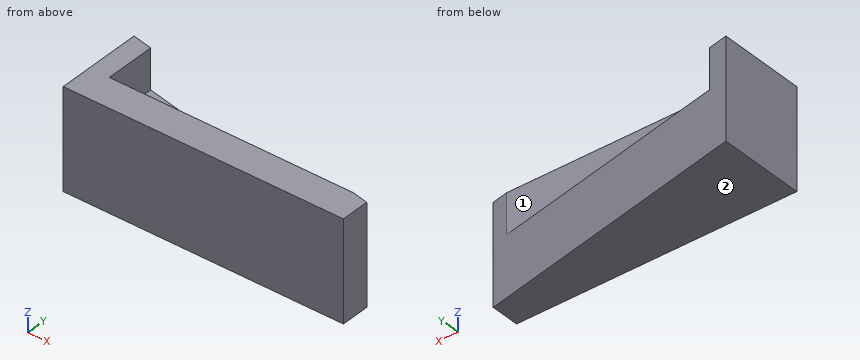
from build123d import *

# Parameters (mm, degrees)
F1_DEPTH = 15
F3_DEPTH = 10
F6_DEPTH = 3
F8_DEPTH = 25


with BuildPart() as f1:
    # F0 (on Top) → F1 (new body)
    with BuildSketch(Plane.XY):
        Polygon((60, 12.5), (0, 0), (60, 0), align=None)
        Polygon((60, 12.5), (60, 0), (90, 0), (90, 18.75), align=None)
    extrude(amount=F1_DEPTH)

    # F2 (on face) → F3 (join)
    with BuildSketch(Plane.XY.offset(15)):
        Polygon((0, 0), (90, 0), (90, 18.75), (85.0000008941, 17.7083335196), (85.0000008941, 5), (24, 5), align=None)
    extrude(amount=F3_DEPTH)


with BuildPart() as f4_1:
    # F4: instance of F1
    add(f1.part.mirror(Plane.YZ))

    # F6 (add): a face of the model
    f6_faces = [f4_1.faces().sort_by_distance(p)[0] for p in [
        (-45, 0, 12.5),
    ]]
    extrude(f6_faces, amount=F6_DEPTH)

    # F7 (on face) → F8 (cut, through all)
    with BuildSketch(Plane.XY.offset(25)):
        Polygon((-20, -3), (0, -3), (0, 0), (-20, 4.1666666667), align=None)
    extrude(amount=-F8_DEPTH, mode=Mode.SUBTRACT)


solid = f4_1.part
Verification items for the finished model (mm, model axes). Face numbers are marked on the shaded views. A direction names the side the tool comes from. Give positions to 0.01 mm unless a question says otherwise; leave off trailing zeros. Loops run counter-clockwise (first coordinate to the right, second up) from the corner with the lowest first, then second, coordinate; pieces in that order, holes last. Notation, with made-up numbers: (53, 69.5) - (102, 69.5) arc R12 cw to (102, 82.5) - close; hole circle Ø5 at (49.5, -17). An arc over 180 degrees is marked (long way). Write item = value, one per line. Start each with the question number.
Q1. Cross-section at D-D, the plane z = 5.75. Enter the section's corners in (x, y).
Q2. Thickness scan on line 1 (Z direction, x = -67, y = 11.75); line 2 (X direction, y = 12.25, z = 17.5); line 3 (Y direction, x = -51.5, z = 21.5). Record the ranges inside material, lowest first.
Q3. Cross-section at A-A, the plane z = 15.75. Enter the section's corners in (x, y).
Q4. Tool access check on the marked faces 1 and 2. Record the directions out of +Z, -Z, +X, -X, +Y, -Y that give a thin tool (end or side, any length) a straight path to the whole face; none if there is none.
Q5. Cross-section at B-B, the plane y = 8.75. Enter the section's corners in (x, z), and give its area (3 significant figures).
Q6. Depth check by flat-ended pin: P1, Ø1.5, axis at x = -32, z = 21.5, coming from the +Y side; P2, Ø3, axis at y = 7.5, z = 19.5, coming from the +X side; P3, Ø4, axis at x = -59.5, y = 14.5, coming from the +Z side; P4, Ø1, axis at x = -67.5, y = 9.5, coming from the +Z side. Enter the tip coordinate at first touch or a pass-through.
Q7. Cross-section at C-C, the plane x = -78. Enter the section's corners in (y, z), and give its area (3 significant figures).
Answer key:
q1.outline = (-90, -3) - (-20, -3) - (-20, 4.17) - (-90, 18.75) - close
q2.line_1 = 0 to 15
q2.line_2 = -90 to -85
q2.line_3 = -3 to 5
q3.outline = (-90, -3) - (-20, -3) - (-20, 4.17) - (-24, 5) - (-85, 5) - (-85, 17.71) - (-90, 18.75) - close
q4.face_1 = +Z, +X, +Y
q4.face_2 = -Z, +X, -X, +Y, -Y
q5.outline = (-90, 0) - (-42, 0) - (-42, 15) - (-85, 15) - (-85, 25) - (-90, 25) - close
q5.area = 770 mm^2
q6.P1 = 5
q6.P2 = -85
q6.P3 = through
q6.P4 = 15
q7.outline = (-3, 0) - (16.25, 0) - (16.25, 15) - (5, 15) - (5, 25) - (-3, 25) - close
q7.area = 369 mm^2
